Here's how the part is built. I have some questions about the finished solid (model axes, mm). A direction names the side the tool comes from. Round coordinates to 2 decimals unless told otherwise and drop trailing zeros. Order: outer loops, then holes, each group sorted by start corner. A loop starts at its lowest first (then second) coordinate and runs counter-clockwise, first axis right, second up. Notation, with made-up numbers: (-37, 66.5) - (7, 66.5) arc R20 ccw to (7, 91.5) - close; hole circle Ø1 at (12, 44). An arc over 180 degrees is marked (long way). One line per item, written item: value.
from build123d import *

# Parameters (mm, degrees)
F0_W      = 100.5620509386
F0_H      = 102.8282381594
F1_DEPTH  = 9
F2_R      = 3.4110604721
F3_DEPTH  = 2
F9_DEPTH  = 2
F17_DEPTH = 2
F19_DEPTH = 2
F21_DEPTH = 2


# Not quite as in the source:
# - the program builds the solid bodies; features that only make, move or delete a surface that nothing else refers to are left out


with BuildPart() as f1:
    # F0 (on Top) → F1 (new body)
    with BuildSketch(Plane.XY):
        with Locations((2.2661872208, -9.3480218202)):
            Rectangle(F0_W, F0_H)
    extrude(amount=F1_DEPTH)

    # F2 (on face) → F3 (join)
    with BuildSketch(Plane.XY.offset(9)):
        with Locations((4.6740118414, -33.5678942502)):
            Circle(F2_R)
    extrude(amount=F3_DEPTH)

    # F8 (on face) → F9 (join)
    with BuildSketch(Plane.XY.offset(9)):
        with BuildLine():
            Line((-4.1074641049, -20.5373205245), (2.40785712, -31.0184087486))
            ThreePointArc((2.40785712, -31.0184087486), (3.2003162928, -30.4916050937), (4.1074650362, -30.2042120027))
            Line((4.1074650362, -30.2042120027), (4.1074650362, -16.0049479455))
            Line((4.1074650362, -16.0049479455), (11.1892977729, -16.0049479455))
            Line((11.1892977729, -16.0049479455), (15.155127272, -13.4554868564))
            Line((15.155127272, -13.4554868564), (25.63624084, -13.4554868564))
            Line((25.63624084, -13.4554868564), (32.1515314281, -16.8547667563))
            Line((32.1515314281, -16.8547667563), (52.5472126901, -16.8547667563))
            Line((52.5472126901, -16.8547667563), (52.5472126901, -3.2576438971))
            Line((52.5472126901, -3.2576438971), (32.1515314281, -3.2576438971))
            Line((32.1515314281, -3.2576438971), (25.63624084, -6.8936358156))
            Line((25.63624084, -6.8936358156), (15.5831124042, -6.8936358156))
            Line((15.5831124042, -6.8936358156), (10.3394780308, -3.8241909351))
            Line((10.3394780308, -3.8241909351), (2.9743718915, -3.8241909351))
            Line((2.9743718915, -3.8241909351), (2.9743718915, 5.8071040548))
            Line((2.9743718915, 5.8071040548), (-4.6740109101, 5.8071040548))
            Line((-4.6740109101, 5.8071040548), (-8.0732917413, 0))
            Line((-8.0732917413, 0), (-48.0148382485, 0))
            Line((-48.0148382485, 0), (-48.0148382485, -24.7864220291))
            Line((-48.0148382485, -24.7864220291), (-15.1551263407, -24.7864220291))
            Line((-15.1551263407, -24.7864220291), (-11.1892987043, -20.5373205245))
            Line((-11.1892987043, -20.5373205245), (-4.1074641049, -20.5373205245))
        make_face()
    extrude(amount=F9_DEPTH)

    # F16 (on face) → F17 (join)
    with BuildSketch(Plane.XY.offset(9)):
        Polygon((-14.1233374194, 17.1550600206), (-11.7558455095, 9.2063853517), (0, 13.1722129881), (-2.6493984959, 21.0257866344), align=None)
    extrude(amount=F17_DEPTH)

    # F18 (on face) → F19 (join)
    with BuildSketch(Plane.XY.offset(9)):
        Polygon((0, 30.7351611555), (-4.6740109101, 35.2675393224), (-12.9274129612, 26.4375342768), (-8.4126724433, 22.0596002612), align=None)
    extrude(amount=F19_DEPTH)

    # F20 (on face) → F21 (join)
    with BuildSketch(Plane.XY.offset(9)):
        Polygon((-18.8376810402, 35.5508103967), (-10.3394789621, 38.9500930905), (-9.7729321569, 42.0660972595), (-21.4437972133, 42.0660972595), align=None)
    extrude(amount=F21_DEPTH)


solid = f1.part
Q1. Which directions (+Z, -Z, +X, -X, +Y, -Y) give clear straight access to the entire face, cutting with the end or side of a thin tool? Please do faces 4 (the flat face through (-5.96, 11.16, 9.99)), 5 (the flat face through (-20.159, 38.854, 9.986)), 6 (the flat face through (-7, 15, 11)), 7 (the flat face through (-2.304, 32.97, 9.986)), 8 (the flat face through (13, -5.38, 9.99)).
Results list:
face 4: +Z, +X
face 5: +Z, -X
face 6: +Z, +X, -X, +Y, -Y
face 7: +Z, +X, +Y
face 8: +Z, +Y
Q2. If I drill on line 1 along X through (y, z) = (-20, 9.75); line 2 along Z through (x, y) = (-32, 6); line 3 along X through (y, z) = (5.5, 9.5), over which ranges is the centre line in solid material (lowest first)?
Results list:
line 1: -48.01 to 4.11
line 2: 0 to 9
line 3: -4.85 to 2.97
Q3. If we section it at B-B, the plane x = 22: Please give me the cut outline in (y, z), then the cut area to 3 significant figures.
Results list:
outline: (-60.76, 0) - (42.07, 0) - (42.07, 9) - (-6.89, 9) - (-6.89, 11) - (-13.46, 11) - (-13.46, 9) - (-60.76, 9) - close
area: 939 mm²
Q4. We'd pull the mould along Y, two halves only. Please class faces 1 (the flat face through (52.547, -10, 4)), 2 (the flat face through (28.94, -5.05, 9.99)), 3 (the flat face through (-14.648, 37.227, 9.986)): released by +Y, released by -Y, zero draft, split by the parting line, or undercut.
Results list:
face 1: zero draft
face 2: released by +Y
face 3: undercut
Q5. If we section it at A-A, the plane x = 44.5: Please give me the cut outline in (y, z), then the cut area to 3 significant figures.
Results list:
outline: (-60.76, 0) - (42.07, 0) - (42.07, 9) - (-3.26, 9) - (-3.26, 11) - (-16.85, 11) - (-16.85, 9) - (-60.76, 9) - close
area: 953 mm²
Q6. Will these pins go through, and if not, where does the flat tip stop? pin 1 (1.6 mm diameter, centred on x = -27, z = 10, fed in from -Y); pin 2 (1.6 mm diameter, centred on x = -2.5, z = 10, fed in from +Y); pin 3 (1 mm diameter, centred on x = 18, z = 10.5, fed in from -Y).
Results list:
pin 1: y = -24.79
pin 2: y = 33.94
pin 3: y = -13.46
